For this review, use the dimensioned drawing (mm, ordinates from the lowest corner) and the shaded views. Coordinates: 2 decimals unless noted, no trailing zeros. Loops run counter-clockwise (first coordinate to the right, second up) from the corner with the lowest first, then second, coordinate; pieces in that order, holes last. Notation, with made-up numbers: (25, 83) - (39, 83) arc R25 ccw to (39, 122) - close; hole circle Ø2 at (-13, 74). An arc over 180 degrees is marked (long way). Use a Markdown table: item, result. Add a question column.
1) Add section B-B, the plane z = 6.25. Give the boundary of the cut face in (x, y).
2) Clearance check with a flat-ended pin moving along its axis: pin 1 (1.5 mm diameter, centred on x = 2.5, z = 5, fed in from +Y). State where the tip first meets the part, or that it passes through.
3) The part is to be moulded in two halves that separate along Z. For the marked faces 1 and 2, say which applies: pulls with the +Z half, pulls with the -Z half, needs draft (parallel to the pull), parting line crosses it, or undercut.
4) Add section A-A, the plane x = 5. Give the boundary of the cut face in (y, z).
5) To check wall thickness, follow L1, parallel to Z at x = 6.75, y = 0.8; L2, parallel to X at y = 0.8, z = 3; L3, parallel to Y at x = 3.25, z = 6. State the ranges of each line that lie inside material, in increasing order. Write a range as [from, to].
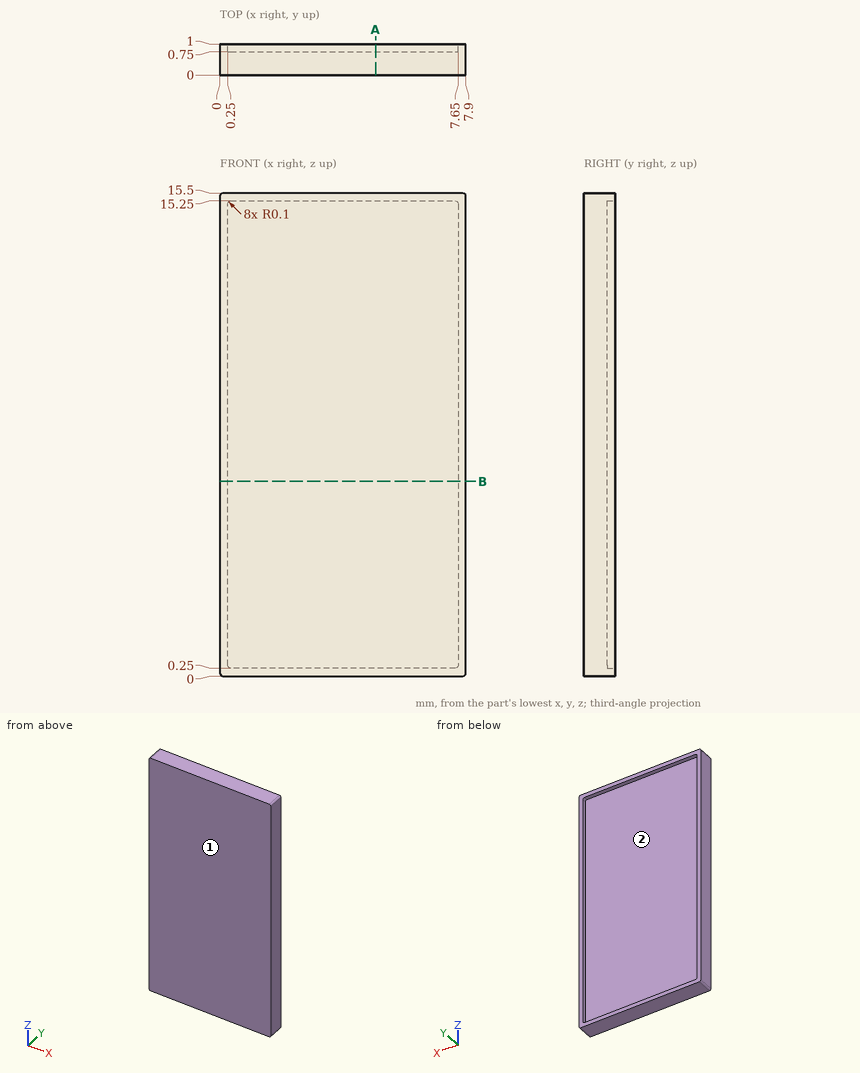
From the geometry:
| question | item | result |
|---|---|---|
| 1 | outline | (0, 0) - (7.9, 0) - (7.9, 1) - (7.65, 1) - (7.65, 0.75) - (0.25, 0.75) - (0.25, 1) - (0, 1) - close |
| 2 | pin 1 | stops at y = 0.75 |
| 3 | face 1 | needs draft |
| 3 | face 2 | undercut |
| 4 | outline | (0, 0) - (1, 0) - (1, 0.25) - (0.75, 0.25) - (0.75, 15.25) - (1, 15.25) - (1, 15.5) - (0, 15.5) - close |
| 5 | L1 | z = [0, 0.25], [15.25, 15.5] |
| 5 | L2 | x = [0, 0.25], [7.65, 7.9] |
| 5 | L3 | y = [0, 0.75] |
